Geometry: see drawing. Coordinates: mm, zero at the bounding-box minimum. A direction names the side the tool comes from. Give positions to 0.01 mm unless a question says otherwise; leave off trailing zeros. Loops run counter-clockwise (first coordinate to the right, second up) from the corner with the lowest first, then second, coordinate; pieces in that order, holes last. Notation, with made-up numbers: M 8.25,-15.75 L 62.25,-15.75 A29 cw 62.25,10.25 Z; hole C -27.5,53 d3. An arc over 180 degrees is marked long. Return JSON: item names as keys, results as strings. Group by question number.
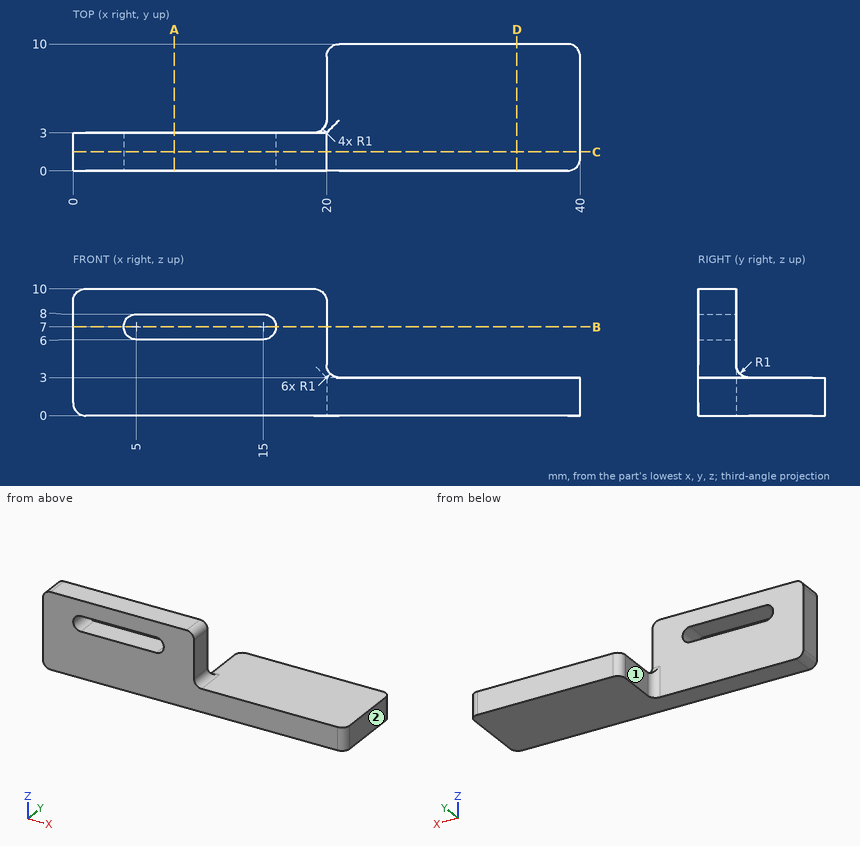
Item 1: Section C-C, the plane y = 1.5. Return loops of the section in (x, z), then the cut area to 3 significant figures.
Item 2: Section B-B, the plane z = 7. Return loops of the section in (x, y), then the cut area to 3 significant figures.
Item 3: Section D-D, the plane x = 35. Return loops of the section in (y, z), then the cut area to 3 significant figures.
Item 4: Reachability of the marked faces 1 and 2 from +Z, -Z, +X, -X, +Y, -Y: full face, straight path, thin tool, end or side. Return the list, or none.
Item 5: Material intervals for line 1 (Z direction, x = 13, y = 2); line 2 (Y direction, x = 17.5, z = 3.25), sorted ascending. Write a range as from..to.
Item 6: First-contact query: pin 1 Ø5 at (y, z) = (6, 4.5) entering from -X; pin 2 Ø3.5 at (y, z) = (2, 6.5) entering from +X; pin 3 Ø3 at (x, y) = (27.5, 3) entering from +Z. Flat tips, straight axial feed; report the tip coordinate or a pass-through.
Item 7: Section A-A, the plane x = 8. Return loops of the section in (y, z).
Answer below:
{
 "1": {"outline": "M 0,1 A1 ccw 1,0 L 40,0 L 40,3 L 21,3 A1 cw 20,4 L 20,9 A1 ccw 19,10 L 1,10 A1 ccw 0,9 Z; hole M 5,6 L 15,6 A1 ccw 15,8 L 5,8 A1 ccw Z", "area": "236 mm^2"},
 "2": {"outline": "M 0,0 L 4,0 L 4,3 L 0,3 Z; M 16,0 L 20,0 L 20,3 L 16,3 Z", "area": "24.0 mm^2"},
 "3": {"outline": "M 0,0 L 10,0 L 10,3 L 0,3 Z", "area": "30.0 mm^2"},
 "4": {"face 1": "+Z, -Z, -X, +Y", "face 2": "+Z, -Z, +X, +Y, -Y"},
 "5": {"line 1": "0..6, 8..10", "line 2": "0..3"},
 "6": {"pin 1": "x = 20", "pin 2": "x = 20", "pin 3": "z = 3"},
 "7": {"outline": "M 0,0 L 3,0 L 3,6 L 0,6 Z; M 0,8 L 3,8 L 3,10 L 0,10 Z"}
}
